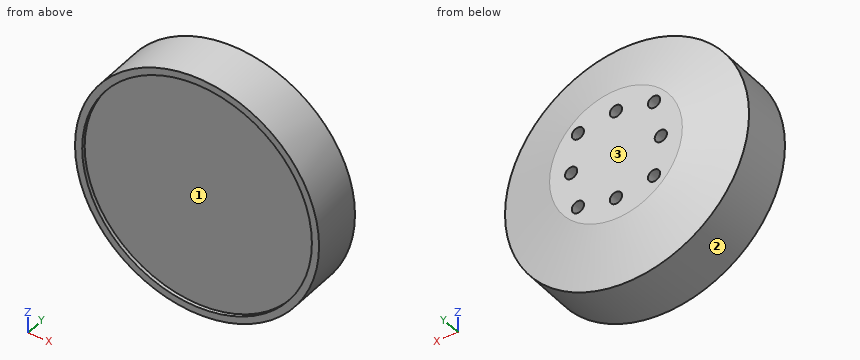
from build123d import *

# Parameters (mm, degrees)
M3_CLEARANCE_HOLE1_D     = 3.4
M3_CLEARANCE_HOLE1_DEPTH = 4
M3_CLEARANCE_HOLE1_TIP   = 1.021463052
SKETCH5_R                = 32
CUT_EXTRUDE1_DEPTH       = 1


with BuildPart() as part:
    # Sketch1 → Revolve1 (revolve)
    with BuildSketch(Plane.XY, mode=Mode.PRIVATE) as revolve1_sk:
        Polygon((0, -9.55), (0, 9.55), (-18.5, 9.55), (-34, 5.05), (-34, -9.55), align=None)
    revolve(revolve1_sk.sketch.rotate(Axis((0, -9.55, 0), (0, 1, 0)), 180), axis=Axis((0, -9.55, 0), (0, 1, 0)))

    # M3 Clearance Hole1
    with Locations(Plane(origin=(0, 9.55, 0), x_dir=(1, 0, 0), z_dir=(0, 1, 0))):
        with Locations((-10.606601718, 10.606601718), (0, 12.5), (10.606601718, 10.606601718), (12.5, 0), (10.606601718, -10.606601718), (-10.606601718, -10.606601718), (-12.5, 0), (0, -12.5)):
            Hole(M3_CLEARANCE_HOLE1_D / 2, depth=M3_CLEARANCE_HOLE1_DEPTH)
            with Locations((0, 0, -(M3_CLEARANCE_HOLE1_DEPTH + M3_CLEARANCE_HOLE1_TIP / 2))):  # 118° drill point
                Cone(0, M3_CLEARANCE_HOLE1_D / 2, M3_CLEARANCE_HOLE1_TIP, mode=Mode.SUBTRACT)

    # Sketch5 → Cut-Extrude1 (cut)
    with BuildSketch(Plane.XZ.offset(9.55)):
        Circle(SKETCH5_R)
    extrude(amount=-CUT_EXTRUDE1_DEPTH, mode=Mode.SUBTRACT)


solid = part.part
Verification items for the finished model (mm, model axes). Face numbers are marked on the shaded views. Round coordinates to 2 decimals unless told otherwise and drop trailing zeros. Use a Markdown table: item, result. Add a question column.
1. Release check for a two-part mould opening along Z. For the marked faces 1, 2 and 3 record: released by +Z, released by -Z, zero draft, split by the parting line, or undercut.
2. Thickness scan on probe 1 along Y at (x, z) = (-0.5, -9.5); probe 2 along Z at (x, y) = (0, -9.3); probe 3 along Z at (x, y) = (13.5, -5.25). Record the ranges inside material, lowest first. Write a range as [from, to].
3. Section check A-A, the plane y = 6.5. Give the number of separate pieces and of enclosed holes in the cut face, plus the area to 3 significant figures.
4. Gauge pin test, flat ends, axial feed: pin 1 (3 mm diameter, centred on x = 2, y = 2.5, fed in from -Z); pin 2 (2 mm diameter, centred on x = -12.5, z = 0, fed in from -Y); pin 3 (1.5 mm diameter, centred on y = -4.5, z = 25.5, fed in from -X). Record the tip position at first contact, or that the pin passes through.
Checks:
| question | item | result |
|---|---|---|
| 1 | face 1 | undercut |
| 1 | face 2 | split by the parting line |
| 1 | face 3 | zero draft |
| 2 | probe 1 | y = [-8.55, 9.55] |
| 2 | probe 2 | z = [-34, -32], [32, 34] |
| 2 | probe 3 | z = [-31.2, 31.2] |
| 3 | separate pieces | 1 |
| 3 | enclosed holes | 8 |
| 3 | area | 2,570 mm^2 |
| 4 | pin 1 | stops at z = -34 |
| 4 | pin 2 | stops at y = -8.55 |
| 4 | pin 3 | stops at x = -23.31 |
